from build123d import *

# Parameters (mm, degrees)
F0_W        = 119.634
F0_H        = 5.9182
F0_W_2      = 5.715
F0_H_2      = 4.9022
F1_DEPTH    = 76.2
F1_FACE_W   = 119.634
F1_FACE_H   = 5.9182
F1_FACE_W_2 = 5.715
F1_FACE_H_2 = 4.9022
F2_DEPTH    = 25.4


with BuildPart() as f1:
    # F0 (on Top) → F1 (new body)
    with BuildSketch(Plane.XY):
        with Locations((59.817, 2.9591)):
            Rectangle(F0_W, F0_H)
        with Locations((3.1115, 2.9591)):
            Rectangle(F0_W_2, F0_H_2, mode=Mode.SUBTRACT)
        with Locations((9.0805, 2.9591)):
            Rectangle(F0_W_2, F0_H_2, mode=Mode.SUBTRACT)
        with Locations((15.0495, 2.9591)):
            Rectangle(F0_W_2, F0_H_2, mode=Mode.SUBTRACT)
        with Locations((21.0185, 2.9591)):
            Rectangle(F0_W_2, F0_H_2, mode=Mode.SUBTRACT)
        with Locations((26.9875, 2.9591)):
            Rectangle(F0_W_2, F0_H_2, mode=Mode.SUBTRACT)
        with Locations((32.9565, 2.9591)):
            Rectangle(F0_W_2, F0_H_2, mode=Mode.SUBTRACT)
        with Locations((38.9255, 2.9591)):
            Rectangle(F0_W_2, F0_H_2, mode=Mode.SUBTRACT)
        with Locations((44.8945, 2.9591)):
            Rectangle(F0_W_2, F0_H_2, mode=Mode.SUBTRACT)
        with Locations((50.8635, 2.9591)):
            Rectangle(F0_W_2, F0_H_2, mode=Mode.SUBTRACT)
        with Locations((56.8325, 2.9591)):
            Rectangle(F0_W_2, F0_H_2, mode=Mode.SUBTRACT)
        with Locations((62.8015, 2.9591)):
            Rectangle(F0_W_2, F0_H_2, mode=Mode.SUBTRACT)
        with Locations((68.7705, 2.9591)):
            Rectangle(F0_W_2, F0_H_2, mode=Mode.SUBTRACT)
        with Locations((74.7395, 2.9591)):
            Rectangle(F0_W_2, F0_H_2, mode=Mode.SUBTRACT)
        with Locations((80.7085, 2.9591)):
            Rectangle(F0_W_2, F0_H_2, mode=Mode.SUBTRACT)
        with Locations((86.6775, 2.9591)):
            Rectangle(F0_W_2, F0_H_2, mode=Mode.SUBTRACT)
        with Locations((92.6465, 2.9591)):
            Rectangle(F0_W_2, F0_H_2, mode=Mode.SUBTRACT)
        with Locations((98.6155, 2.9591)):
            Rectangle(F0_W_2, F0_H_2, mode=Mode.SUBTRACT)
        with Locations((104.5845, 2.9591)):
            Rectangle(F0_W_2, F0_H_2, mode=Mode.SUBTRACT)
        with Locations((110.5535, 2.9591)):
            Rectangle(F0_W_2, F0_H_2, mode=Mode.SUBTRACT)
        with Locations((116.5225, 2.9591)):
            Rectangle(F0_W_2, F0_H_2, mode=Mode.SUBTRACT)
    extrude(amount=F1_DEPTH)

    # F1_face (on face) → F2 (join)
    with BuildSketch(Plane(origin=(59.817, 2.9591, 0), x_dir=(1, 0, 0), z_dir=(0, 0, -1))):
        Rectangle(F1_FACE_W, F1_FACE_H)
        with Locations((-56.7055, 0)):
            Rectangle(F1_FACE_W_2, F1_FACE_H_2, mode=Mode.SUBTRACT)
        with Locations((-50.7365, 0)):
            Rectangle(F1_FACE_W_2, F1_FACE_H_2, mode=Mode.SUBTRACT)
        with Locations((-44.7675, 0)):
            Rectangle(F1_FACE_W_2, F1_FACE_H_2, mode=Mode.SUBTRACT)
        with Locations((-38.7985, 0)):
            Rectangle(F1_FACE_W_2, F1_FACE_H_2, mode=Mode.SUBTRACT)
        with Locations((-32.8295, 0)):
            Rectangle(F1_FACE_W_2, F1_FACE_H_2, mode=Mode.SUBTRACT)
        with Locations((-26.8605, 0)):
            Rectangle(F1_FACE_W_2, F1_FACE_H_2, mode=Mode.SUBTRACT)
        with Locations((-20.8915, 0)):
            Rectangle(F1_FACE_W_2, F1_FACE_H_2, mode=Mode.SUBTRACT)
        with Locations((-14.9225, 0)):
            Rectangle(F1_FACE_W_2, F1_FACE_H_2, mode=Mode.SUBTRACT)
        with Locations((-8.9535, 0)):
            Rectangle(F1_FACE_W_2, F1_FACE_H_2, mode=Mode.SUBTRACT)
        with Locations((-2.9845, 0)):
            Rectangle(F1_FACE_W_2, F1_FACE_H_2, mode=Mode.SUBTRACT)
        with Locations((2.9845, 0)):
            Rectangle(F1_FACE_W_2, F1_FACE_H_2, mode=Mode.SUBTRACT)
        with Locations((8.9535, 0)):
            Rectangle(F1_FACE_W_2, F1_FACE_H_2, mode=Mode.SUBTRACT)
        with Locations((14.9225, 0)):
            Rectangle(F1_FACE_W_2, F1_FACE_H_2, mode=Mode.SUBTRACT)
        with Locations((20.8915, 0)):
            Rectangle(F1_FACE_W_2, F1_FACE_H_2, mode=Mode.SUBTRACT)
        with Locations((26.8605, 0)):
            Rectangle(F1_FACE_W_2, F1_FACE_H_2, mode=Mode.SUBTRACT)
        with Locations((32.8295, 0)):
            Rectangle(F1_FACE_W_2, F1_FACE_H_2, mode=Mode.SUBTRACT)
        with Locations((38.7985, 0)):
            Rectangle(F1_FACE_W_2, F1_FACE_H_2, mode=Mode.SUBTRACT)
        with Locations((44.7675, 0)):
            Rectangle(F1_FACE_W_2, F1_FACE_H_2, mode=Mode.SUBTRACT)
        with Locations((50.7365, 0)):
            Rectangle(F1_FACE_W_2, F1_FACE_H_2, mode=Mode.SUBTRACT)
        with Locations((56.7055, 0)):
            Rectangle(F1_FACE_W_2, F1_FACE_H_2, mode=Mode.SUBTRACT)
    extrude(amount=F2_DEPTH)


solid = f1.part
Input: part model. Units: mm. Frame: model coordinates. Round coordinates to 2 decimals unless told otherwise and drop trailing zeros. Write each loop counter-clockwise with the first axis right and the second up, starting at its lowest first coordinate (ties: lowest second). Pieces come first, ordered by that corner, then holes.
1) Cut plane B-B (y = 1.45). Count the separate pieces of the cut face and the enclosed holes in it, then the cut area to 3 significant figures.
2) Cut plane A-A (x = 22.5). Return the cut outline in (y, z).
3) Draft query along Y for faces 1 (the flat face through (87, 0.508, 26)), 2 (the flat face through (111, 5.41, 26)), 3 (the flat face through (119.634, 3, 26)). Return one class per face: pulls with the +Y half, pulls with the -Y half, needs draft (parallel to the pull), parting line crosses it, or undercut.
4) Ray query, L1, parallel to Y at x = 102, z = 20.5. Return the intervals inside material, ascending.
Geometry says:
1. separate pieces: 21
1. enclosed holes: 0
1. area: 542 mm2
2. outline: (0, -25.4) - (0.51, -25.4) - (0.51, 76.2) - (0, 76.2) - close; (5.41, -25.4) - (5.92, -25.4) - (5.92, 76.2) - (5.41, 76.2) - close
3. face 1: undercut
3. face 2: undercut
3. face 3: needs draft
4. L1: y = 0 to 0.51, 5.41 to 5.92
